Autodesk Inventor part; units mm, degrees
ref_plane "Płaszczyzna konstrukcyjna1" through (30, -2.5, -105) normal (1, 0, 0) x (0, 0, -1)
ref_plane "Płaszczyzna konstrukcyjna2" through (-23, -2.5, 105) normal (-1, 0, 0) x (0, 0, 1)
ref_plane "YZ Plane" through (0, 0, 0) normal (1, 0, 0) x (0, 1, 0)
sketch "Szkic1" plane through (0, 0, 0) normal (0, 1, 0) x (-1, 0, 0)
  line L0 (-35, 105) -> (35, 105)
  line L1 (35, 105) -> (35, -105)
  line L2 (35, -105) -> (-35, -105)
  line L3 (-35, -105) -> (-35, 105)
  line L4 (-35, 105) -> (35, -105) construction
  line L5 (35, 105) -> (-35, -105) construction
  line L6 (-35, 105) -> (-25, 105)
  line L7 (-30, 105) -> (-30, 90)
  line L8 (35, 105) -> (28, 105)
  line L9 (28, 105) -> (28, -105)
  line L10 (35, -105) -> (28, -105)
  circle A0 centre (-30, 90) radius 2.15
  circle A1 centre (-30, 45) radius 2.15
  circle A2 centre (-30, 0) radius 2.15
  circle A3 centre (-30, -45) radius 2.15
  circle A4 centre (-30, -90) radius 2.15
  line L11 (-35, 105) -> (-35, 55)
  line L12 (-35, 55) -> (-6, 55)
  line L13 (-20, 79) -> (8, 79)
  line L14 (8, 79) -> (8, 31)
  line L15 (8, 31) -> (-20, 31)
  line L16 (-20, 31) -> (-20, 79)
  line L17 (-20, 79) -> (8, 31) construction
  line L18 (8, 79) -> (-20, 31) construction
  point P0 (0, 0)
  point P1 (0, 0)
  dimension "d4" = 70
  dimension "d5" = 210
  dimension "d6" = 10
  dimension "d7" = 15
  dimension "d8" = 7
  dimension "d9" = 4.3
  dimension "d10" = 45
  dimension "d12" = 50
  dimension "d13" = 29
  dimension "d14" = 28
  dimension "d15" = 48
extrude "Wyciągnięcie proste1" add sketch "Szkic1" along normal mid plane 5 contours L0 L9 L2 L3
ref_plane "Płaszczyzna konstrukcyjna1" through (30, -2.5, -105) normal (1, 0, 0) x (0, 0, -1)
ref_plane "Płaszczyzna konstrukcyjna2" through (-23, -2.5, 105) normal (-1, 0, 0) x (0, 0, 1)
sketch "Szkic3" plane through (-23, -2.5, 105) normal (-1, 0, 0) x (0, 0, 1)
  line L0 (-224.7917, 43.2301) -> (-14.7917, 43.2301)
  line L1 (-224.7917, 43.2301) -> (-14.7917, 43.2301)
  line L2 (-119.7917, 43.2301) -> (-119.7917, 58.2301)
  circle A0 centre (-119.7917, 58.2301) radius 2.15
  line L3 (-119.7917, 60.3801) -> (-119.7917, 63.3801)
  line L4 (-150.7917, 43.2301) -> (-198.7917, 43.2301)
  arc A1 (-119.7917, 63.3801) -> (-154.3457, 43.2301) centre (-119.6183, 23.3805) ccw
  arc A2 (-85.2378, 43.2301) -> (-119.7917, 63.3801) centre (-119.9652, 23.3805) ccw
  line L5 (-154.3457, 43.2301) -> (-85.2378, 43.2301)
  line L6 (-210, 0) -> (-210, 5)
  line L7 (-210, 0) -> (0, 0)
  line L8 (-210, 0) -> (0, 0)
  line L9 (-105, 0) -> (-105, -15)
  circle A3 centre (-105, -15) radius 2.15
  line L10 (-105, -17.15) -> (-105, -20.15)
  arc A4 (-139.554, 0) -> (-105, -20.15) centre (-104.8266, 19.8496) ccw
  arc A5 (-105, -20.15) -> (-70.446, 0) centre (-105.1734, 19.8496) ccw
  line L11 (-70.446, 0) -> (-139.554, 0)
  point P0 (-105, 2.5)
  point P1 (-119.7917, 40.7301)
  point P2 (-70.446, 0)
  point P3 (-139.554, 0)
  dimension "d26" = 4.3
  dimension "d31" = 4.3
  dimension "d25" = 15
  dimension "d27" = 3
  dimension "d28" = 40
  dimension "d29" = 40
  dimension "d30" = 15
  dimension "d32" = 3
  dimension "d33" = 40
  dimension "d34" = 40
extrude "Wyciągnięcie proste2" add sketch "Szkic3" against normal blind 7 contours L7 L9 A3 L10 A4 | L7 A5 L10 A3 L9
properties part number "podstawa_sciana_tyl"
The listing builds one solid part. Answer for the finished solid, in the listing's coordinates (mm). A direction names the side the tool comes from. Give positions to 0.01 mm unless a question says otherwise; leave off trailing zeros. Loops run counter-clockwise (first coordinate to the right, second up) from the corner with the lowest first, then second, coordinate; pieces in that order, holes last. Notation, with made-up numbers: (60.25, 71.25) - (88.25, 71.25) arc R18 ccw to (88.25, 97.25) - close; hole circle Ø10 at (84, -5). An arc over 180 degrees is marked (long way). Return JSON: item names as keys, results as strings. Group by question number.
1. Straight lines are drawn through the part: line 1 (Z direction, x = 30, y = 0.2); line 2 (X direction, y = -2, z = 66); line 3 (Y direction, x = 26.5, z = 7.5). For each, find the intervals that lie inside material, in ascending order. Write a range as [from, to].
2. Find section D-D (x = 30). Write down the section's boundary in (y, z).
3. Given pin 1 Ø6 at (x, z) = (-10.5, -3.5) entering from -Y; pin 2 Ø10 at (y, z) = (-9, -16) entering from +X; pin 3 Ø10 at (y, z) = (-12, -1.5) entering from -X, each flat-ended and moving along its own axis, determine where each tip first touches the part or whether it passes through.
4. Find section A-A (z = -45). Write down the section's boundary in (x, y).
5. Find section C-C (z = 45). Write down the section's boundary in (x, y).
6. Find section B-B (x = 17). Write down the section's boundary in (y, z), then the cut area to 3 significant figures.
7. Determine the mould class of faces 1 (the cylindrical face through (28.84, -0.04, 43.19)), 2 (the cylindrical face through (-19.55, -19.6, -0.47)), 3 (the cylindrical face through (-19.549, -17.056, -20.229)) for opening direction Y: pulls with the +Y half, pulls with the -Y half, needs draft (parallel to the pull), parting line crosses it, or undercut.
8. Which of the six approach directions +Z, -Z, +X, -X, +Y, -Y give full straight-line access (tool end or side, diameter ignored) to faces 4 (the flat face through (35, 0, -1)), 5 (the flat face through (6, 0, 79)), 6 (the flat face through (4, 0, 105)), 7 (the flat face through (-23, -10, 0)), 8 (the flat face through (-16, -10, 0))?
Verdict:
{
 "1": {"line 1": "z = [-105, -92.15], [-87.85, -47.15], [-42.85, -2.15], [2.15, 42.85], [47.15, 87.85], [92.15, 105]", "line 2": "x = [-28, -8], [20, 35]", "line 3": "y = [-2.5, 2.5]"},
 "2": {"outline": "(-2.5, -105) - (2.5, -105) - (2.5, -92.15) - (-2.5, -92.15) - close; (-2.5, -87.85) - (2.5, -87.85) - (2.5, -47.15) - (-2.5, -47.15) - close; (-2.5, -42.85) - (2.5, -42.85) - (2.5, -2.15) - (-2.5, -2.15) - close; (-2.5, 2.15) - (2.5, 2.15) - (2.5, 42.85) - (-2.5, 42.85) - close; (-2.5, 47.15) - (2.5, 47.15) - (2.5, 87.85) - (-2.5, 87.85) - close; (-2.5, 92.15) - (2.5, 92.15) - (2.5, 105) - (-2.5, 105) - close"},
 "3": {"pin 1": "stops at y = -2.5", "pin 2": "stops at x = -16", "pin 3": "stops at x = -23"},
 "4": {"outline": "(-28, -2.5) - (27.85, -2.5) - (27.85, 2.5) - (-28, 2.5) - close; (32.15, -2.5) - (35, -2.5) - (35, 2.5) - (32.15, 2.5) - close"},
 "5": {"outline": "(-28, -2.5) - (-8, -2.5) - (-8, 2.5) - (-28, 2.5) - close; (20, -2.5) - (27.85, -2.5) - (27.85, 2.5) - (20, 2.5) - close; (32.15, -2.5) - (35, -2.5) - (35, 2.5) - (32.15, 2.5) - close"},
 "6": {"outline": "(-2.5, -105) - (2.5, -105) - (2.5, 31) - (-2.5, 31) - close; (-2.5, 79) - (2.5, 79) - (2.5, 105) - (-2.5, 105) - close", "area": "810 mm^2"},
 "7": {"face 1": "needs draft", "face 2": "undercut", "face 3": "pulls with the -Y half"},
 "8": {"face 4": "+Z, -Z, +X, +Y, -Y", "face 5": "+Y, -Y", "face 6": "+Z, +X, -X, +Y, -Y", "face 7": "+Z, -Z, -X, -Y", "face 8": "+Z, -Z, +X, -Y"}
}
